Verification items for the finished model (mm, model axes). A direction names the side the tool comes from. Coordinates: 2 decimals unless noted, no trailing zeros. Write each loop counter-clockwise with the first axis right and the second up, starting at its lowest first coordinate (ties: lowest second). Pieces come first, ordered by that corner, then holes. Notation, with made-up numbers: (-7.75, 0.5) - (51.25, 0.5) arc R26 cw to (51.25, 28.5) - close; hole circle Ø5 at (0.5, -27). An arc over 180 degrees is marked (long way). Answer as CSV lines item,"result". Start each with the question number.
```python
from build123d import *

# Parameters (mm, degrees)
F1_DEPTH = 40


with BuildPart() as f1:
    # F0 (on Top) → F1 (new body)
    with BuildSketch(Plane.XY):
        with BuildLine():
            Line((-80, -20), (-0.902612, -20))
            Line((-0.902612, -20), (0, -20))
            ThreePointArc((0, -20), (7.071068, -17.071068), (10, -10))
            Line((10, -10), (8.5, -10))
            ThreePointArc((8.5, -10), (6.010408, -16.010408), (0, -18.5))
            Line((0, -18.5), (-6.213812, -18.5))
            Line((-6.213812, -18.5), (-39, -18.5))
            Line((-39, -18.5), (-39, -13.5))
            Line((-39, -13.5), (-44.853471, -13.5))
            Line((-44.853471, -13.5), (-44.853471, -10.5))
            Line((-44.853471, -10.5), (-32.853471, -10.5))
            Line((-32.853471, -10.5), (-32.853471, -10))
            Line((-32.853471, -10), (-46.780869, -10))
            Line((-46.780869, -10), (-46.780869, -15))
            Line((-46.780869, -15), (-41, -15))
            Line((-41, -15), (-41, -18.5))
            Line((-41, -18.5), (-59, -18.5))
            Line((-59, -18.5), (-59, -14))
            Line((-59, -14), (-60, -14))
            Line((-60, -14), (-60, -18.5))
            Line((-60, -18.5), (-79, -18.5))
            Line((-79, -18.5), (-79, -16))
            Line((-79, -16), (-80, -16))
            Line((-80, -16), (-80, -18.5))
            Line((-80, -18.5), (-80, -20))
        make_face()
    extrude(amount=F1_DEPTH)


solid = f1.part
```
1. Cross-section at C-C (x = -56.5). Record the cut outline in (y, z), and give its area (3 significant figures).
2. Scan lines: line 1 along X through (y, z) = (-16.5, 34); line 2 along Y through (x, z) = (-46.5, 34); line 3 along Y through (x, z) = (-61, 38). Record each from-to range of solid material in increasing order. Write a range as from..to.
3. Cross-section at A-A (x = -36.5). Record the cut outline in (y, z).
4. Cross-section at B-B (z = 19.5). Record the cut outline in (x, y).
5. Depth check by flat-ended pin: P1, Ø3, axis at x = -32.5, y = -18, coming from the -Z side; P2, Ø1.2, axis at y = -17, z = 24.5, coming from the +X side; P3, Ø1.1, axis at x = -59.5, z = 20, coming from the +Y side; P4, Ø5.5, axis at x = -73.5, z = 28.5, coming from the +Y side. Enter the tip coordinate at first touch or a pass-through.
6. Draft check along X on faces 1 (the face through (-79, -17, 20)), 2 (the face through (-40, -10, 20)), 3 (the face through (6.99, -17.15, 19.72)). Enter one of: pulls with the +X half, pulls with the -X half, needs draft (parallel to the pull), parting line crosses it, or undercut.
7. Access from +Z, -Z, +X, -X, +Y, -Y to the whole of each face (thin tool, end or side, straight path). Record for faces 4 (the face through (-60, -16, 20)), 5 (the face through (-41, -17, 20)), 6 (the face through (-41, -20, 20)).
Completed:
1,outline,"(-20, 0) - (-18.5, 0) - (-18.5, 40) - (-20, 40) - close"
1,area,"60.0 mm2"
2,line 1,"x = -80..-79, -60..-59, -41..-39, 5.48..7.6"
2,line 2,"y = -20..-18.5, -15..-10"
2,line 3,"y = -20..-18.5"
3,outline,"(-20, 0) - (-18.5, 0) - (-18.5, 40) - (-20, 40) - close; (-10.5, 0) - (-10, 0) - (-10, 40) - (-10.5, 40) - close"
4,outline,"(-80, -20) - (0, -20) arc R10 ccw to (10, -10) - (8.5, -10) arc R8.5 cw to (0, -18.5) - (-39, -18.5) - (-39, -13.5) - (-44.85, -13.5) - (-44.85, -10.5) - (-32.85, -10.5) - (-32.85, -10) - (-46.78, -10) - (-46.78, -15) - (-41, -15) - (-41, -18.5) - (-59, -18.5) - (-59, -14) - (-60, -14) - (-60, -18.5) - (-79, -18.5) - (-79, -16) - (-80, -16) - close"
5,P1,"stops at z = 0"
5,P2,"stops at x = 7.68"
5,P3,"stops at y = -14"
5,P4,"stops at y = -18.5"
6,face 1,"undercut"
6,face 2,"needs draft"
6,face 3,"pulls with the +X half"
7,face 4,"+Z, -Z, +Y"
7,face 5,"+Z, -Z"
7,face 6,"+Z, -Z, +X, -X, -Y"
